Check sheet for the drawn part. Datum: minimum x, y, z corner. Units: mm. Give positions to 0.01 mm unless a question says otherwise; leave off trailing zeros. Write each loop counter-clockwise with the first axis right and the second up, starting at its lowest first coordinate (ties: lowest second). Pieces come first, ordered by that corner, then holes. Notation, with made-up numbers: M 66.5,80.25 L 83.5,80.25 A29 ccw 83.5,101.25 Z; hole C 22,22 d11. An arc over 180 degrees is marked long. Write item = value, one per line.
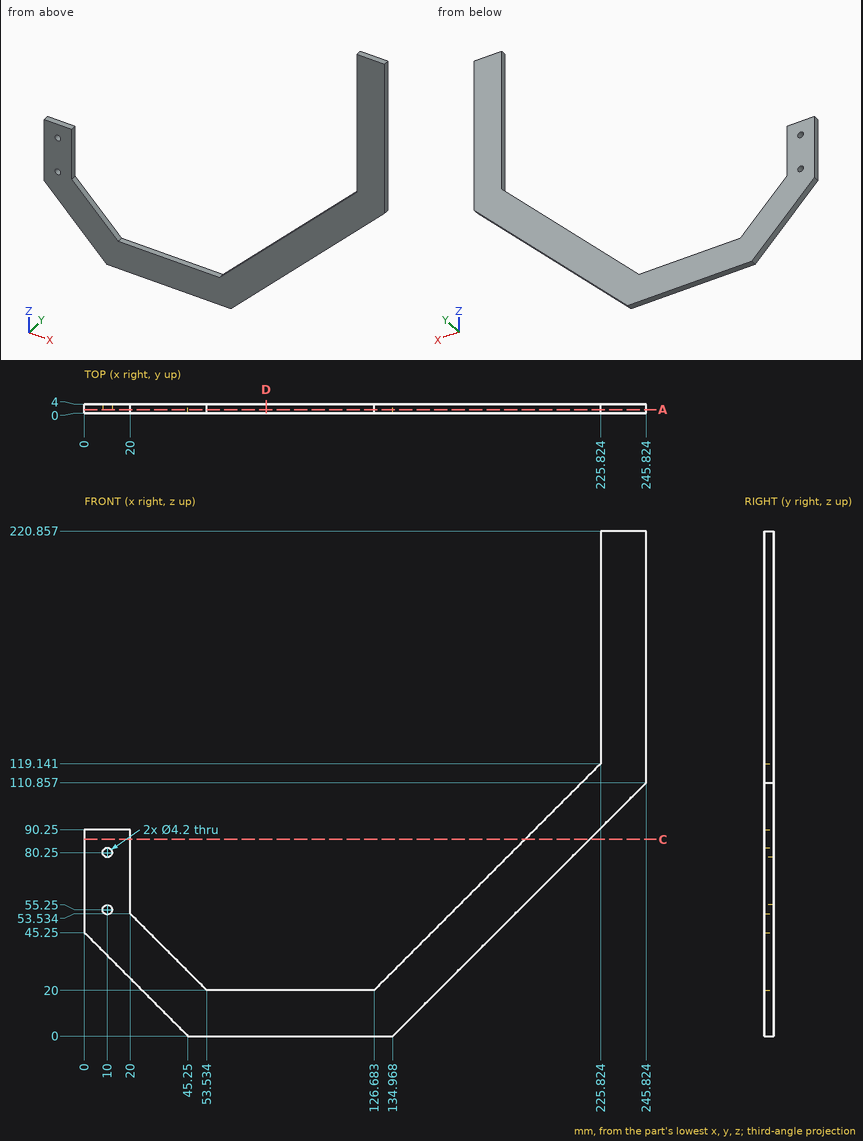
1) Cross-section at C-C on z = 86. Record the boundary of the cut face in (x, y).
From the geometry:
outline = M 0,0 L 20,0 L 20,4 L 0,4 Z; M 192.68,0 L 220.97,0 L 220.97,4 L 192.68,4 Z
2) Cross-section at D-D on x = 79.5. Record the boundary of the cut face in (y, z), plus the area to 3 significant figures.
From the geometry:
outline = M 0,0 L 4,0 L 4,20 L 0,20 Z
area = 80.0 mm^2
3) Depth check by flat-ended pin: P1, Ø1.5, axis at x = 84.5, y = 3, coming from the +Z side; P2, Ø2, axis at x = 52.5, y = 1.5, coming from the +Z side (1 decimal). Enter the tip coordinate at first touch or a pass-through.
From the geometry:
P1 = 20
P2 = 22
4) Cross-section at A-A on y = 1.5. Count the separate pieces of the cut face and the enclosed holes in it, plus the area to 3 significant figures.
From the geometry:
separate_pieces = 1
enclosed_holes = 2
area = 8,620 mm^2
5) Material ranges on probe 1 along X at (y, z) = (2.25, 80.25) (1 decimal); probe 2 along X at (y, z) = (2.8, 142.5) (1 decimal); probe 3 along Z at (x, y) = (58, 3.1), recorded low to high. Write a range as from..to.
From the geometry:
probe_1 = 0..7.9, 12.1..20, 186.9..215.2
probe_2 = 225.8..245.8
probe_3 = 0..20
